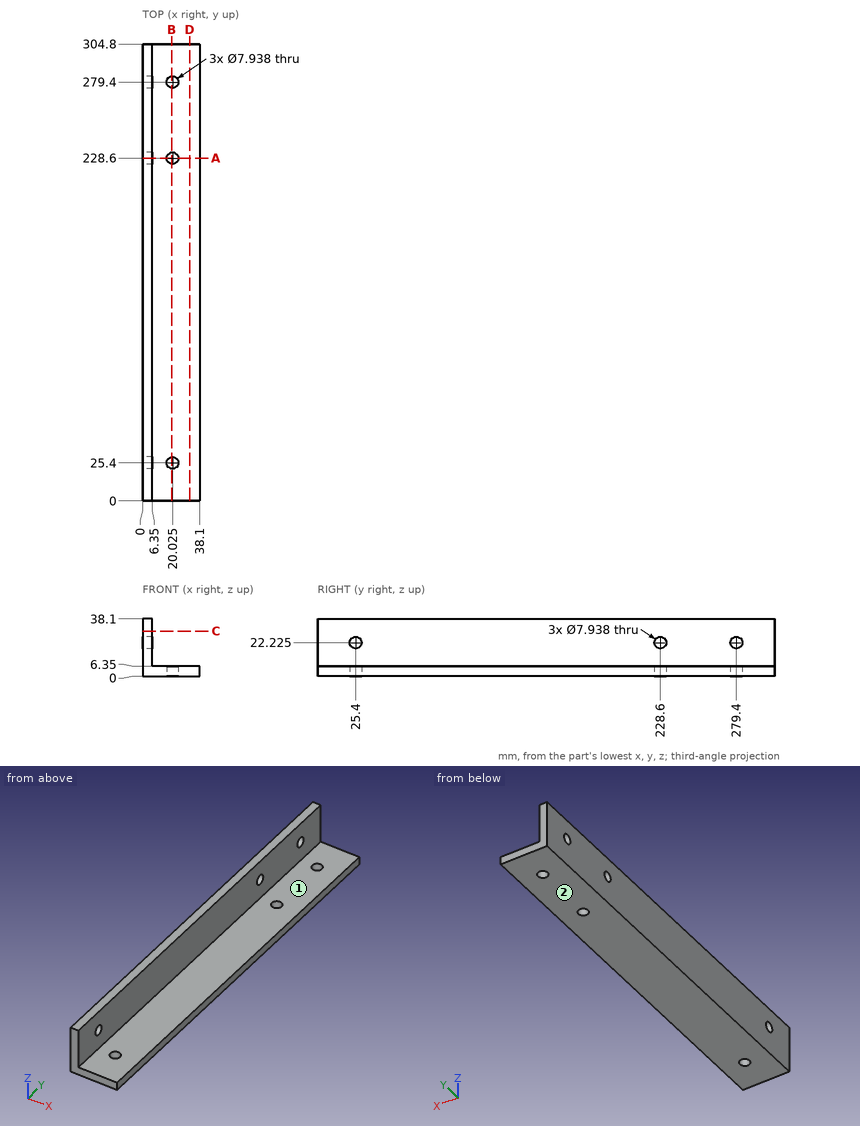
Geometry check sheet. Reference: drawing and pictorial views, mm from the part's lowest x, y, z. A direction names the side the tool comes from. Give positions to 0.01 mm unless a question says otherwise; leave off trailing zeros. Order: outer loops, then holes, each group sorted by start corner. A loop starts at its lowest first (then second) coordinate and runs counter-clockwise, first axis right, second up. Notation, with made-up numbers: M -20,51.25 L -8,51.25 A14 cw -8,77.25 Z; hole C 58,59 d3. An arc over 180 degrees is marked long. Answer as a JSON object with one key per item and string values. Group by question number.
1) Cross-section at C-C (z = 30). Enter the section's corners in (x, y).
2) Scan lines: line 1 along Y through (x, z) = (5.5, 22); line 2 along Z through (x, y) = (2, 228); line 3 along Z through (x, y) = (15.5, 114). Record each from-to range of solid material in increasing order. Write a range as [from, to].
3) Access from +Z, -Z, +X, -X, +Y, -Y to the whole of each face (thin tool, end or side, straight path). Record for the marked faces 1 and 2.
4) Cross-section at A-A (y = 228.6). Give the number of separate pieces and of enclosed holes in the cut face, then the cut area to 3 significant figures.
5) Cross-section at B-B (x = 19.5). Enter the section's corners in (y, z).
6) Depth check by flat-ended pin: pin 1 Ø1 at (y, z) = (268, 17.5) entering from +X; pin 2 Ø10.5 at (x, y) = (20.03, 228.6) entering from +Z. Enter the tip coordinate at first touch or a pass-through.
7) Cross-section at D-D (x = 31.5). Enter the section's corners in (y, z).
Result sheet:
{
 "1": {"outline": "M 0,0 L 6.35,0 L 6.35,304.8 L 0,304.8 Z"},
 "2": {"line 1": "y = [0, 21.44], [29.36, 224.64], [232.56, 275.44], [283.36, 304.8]", "line 2": "z = [0, 18.3], [26.15, 38.1]", "line 3": "z = [0, 6.35]"},
 "3": {"face 1": "+Z, +X, +Y, -Y", "face 2": "-Z, +X, -X, +Y, -Y"},
 "4": {"separate pieces": "3", "enclosed holes": "0", "area": "343 mm2"},
 "5": {"outline": "M 0,0 L 21.47,0 L 21.47,6.35 L 0,6.35 Z; M 29.33,0 L 224.67,0 L 224.67,6.35 L 29.33,6.35 Z; M 232.53,0 L 275.47,0 L 275.47,6.35 L 232.53,6.35 Z; M 283.33,0 L 304.8,0 L 304.8,6.35 L 283.33,6.35 Z"},
 "6": {"pin 1": "stops at x = 6.35", "pin 2": "stops at z = 6.35"},
 "7": {"outline": "M 0,0 L 304.8,0 L 304.8,6.35 L 0,6.35 Z"}
}
